The model under review builds one solid part; all positions refer to its coordinate system, in mm. Face numbers are marked on the shaded views. Coordinates: 2 decimals unless noted, no trailing zeros. Loops run counter-clockwise (first coordinate to the right, second up) from the corner with the lowest first, then second, coordinate; pieces in that order, holes last. Notation, with made-up numbers: (-22, -32) -> (13, -32) arc R14 ccw to (13, -17) -> close; hole circle Ø6 at (59, 15). An arc over 180 degrees is marked (long way). One line per question, with ' | ' between items. Start each with the question number.
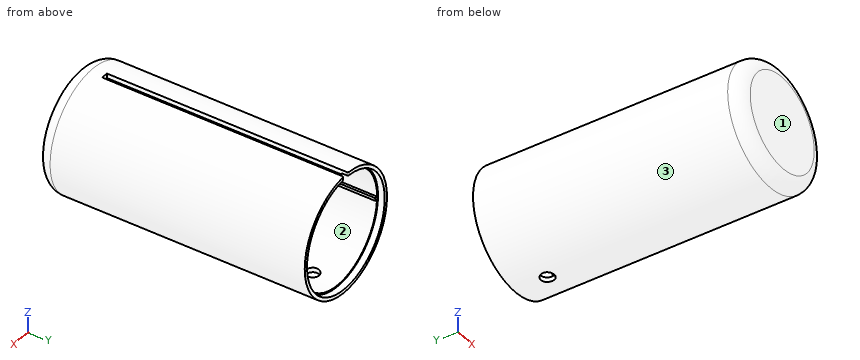
Autodesk Inventor part; units mm, degrees
ref_plane "Work Plane1" through (0, 200, -45) normal (0, 0, -1) x (-1, 0, 0)
ref_plane "YZ Plane" through (0, 0, 0) normal (1, 0, 0) x (0, 1, 0)
ref_plane "XZ Plane" through (0, 0, 0) normal (0, 1, 0) x (-1, 0, 0)
sketch "Sketch1" plane through (0, 0, 0) normal (0, 0, 1) x (1, 0, 0)
  line L0 (0, 0) -> (35, 0)
  line L1 (45, 10) -> (45, 200)
  line L2 (0, 200) -> (0, 0)
  arc A0 (35, 0) -> (45, 10) centre (35, 10) ccw
  line L3 (41.5, 200) -> (41.5, 10)
  arc A1 (35, 3.5) -> (41.5, 10) centre (35, 10) ccw
  line L4 (35, 3.5) -> (0, 3.5)
  line L5 (41.5, 200) -> (45, 200)
  line L6 (0, 3.5) -> (0, 0)
  point P0 (45, 0)
  dimension "d0" = 90
  dimension "d1" = 200
  dimension "d2" = 10
  dimension "d5" = 3.5
  dimension "d6" = 3.5
revolve "Revolution1" add sketch "Sketch1" angle 360 about axis through (0, 200, 0) along (0, -1, 0)
sketch "Sketch2" plane through (0, 200, 0) normal (0, 1, 0) x (1, 0, 0)
  circle A0 centre (0, 0) radius 45 construction
  line L0 (0, 45) -> (0, -45) construction
  line L1 (-45, 0) -> (45, 0) construction
  circle A1 centre (0, 0) radius 45 construction
  circle A2 centre (0, 0) radius 41.5 construction
  circle A3 centre (0, 0) radius 41.5 construction
  circle A4 centre (0, 0) radius 45 construction
  line L2 (0, -41.5) -> (0, -45) construction
  line L3 (-2.5, -45.45) -> (2.5, -45.45)
  line L4 (2.5, -45.45) -> (2.5, -41.05)
  line L5 (2.5, -41.05) -> (-2.5, -41.05)
  line L6 (-2.5, -41.05) -> (-2.5, -45.45)
  line L7 (-2.5, -45.45) -> (2.5, -41.05) construction
  line L8 (2.5, -45.45) -> (-2.5, -41.05) construction
  point P0 (0, -43.25)
  dimension "d8" = 5
  dimension "d9" = 4.4
extrude "Extrusion1" cut sketch "Sketch2" against normal blind 180
fillet "Fillet1" radius 1 2 edges at (-2.5, 200, 43.1776) (2.5, 200, 43.1776)
sketch "Sketch3" plane through (0, 200, 0) normal (0, 1, 0) x (1, 0, 0)
  arc A0 (3.5, -41.3521) -> (-3.5, -41.3521) centre (0, 0) ccw
  circle A1 centre (0, 0) radius 42.5
  circle A2 centre (0, 0) radius 41.5
  point P0 (3.5, -41.3521)
  point P1 (-3.5, -41.3521)
  dimension "d13" = 85
extrude "Extrusion2" cut sketch "Sketch3" against normal blind 5
ref_plane "Work Plane1" through (0, 200, -45) normal (0, 0, -1) x (-1, 0, 0)
sketch "Sketch4" plane through (0, 200, -45) normal (0, 0, -1) x (-1, 0, 0)
  line L0 (-45, 0) -> (45, 0) construction
  line L1 (0, 0) -> (0, -25) construction
  circle A0 centre (0, -25) radius 5
  point P0 (0, -200)
  point P1 (3.5, 0)
  point P2 (-3.5, 0)
  dimension "d16" = 25
  dimension "d17" = 10
extrude "Extrusion3" cut sketch "Sketch4" against normal up to surface
sketch "Sketch5" plane through (0, 195, 0) normal (0, 1, 0) x (1, 0, 0)
  line L0 (2.5, -42.4264) -> (2.5, -41.4246) construction
  arc A0 (2.5, -42.4264) -> (-2.5, -42.4264) centre (0, 0) ccw construction
  line L1 (-2.5, -41.4246) -> (-2.5, -42.4264) construction
  arc A1 (2.5, -41.4246) -> (-2.5, -41.4246) centre (0, 0) ccw
  arc A2 (2.5, -41.4246) -> (-2.5, -41.4246) centre (0, 0) ccw construction
  line L2 (41.5, 0) -> (-41.5, 0) construction
  line L3 (41.5, 0) -> (39.5, 0)
  arc A3 (39.5, 0) -> (39.4459, 2.0673) centre (0, 0) ccw
  line L4 (41.5, 0) -> (39.5, 0)
  line L5 (0, 0) -> (41.5, 0) construction
  line L6 (0, 0) -> (41.4431, 2.1719) construction
  line L7 (41.4431, 2.1719) -> (39.4459, 2.0673)
  line L8 (0, 41.5) -> (0, -41.5) construction
  arc A4 (41.5, 0) -> (41.4431, 2.1719) centre (0, 0) ccw
  arc A5 (-2.5, -41.4246) -> (2.5, -41.4246) centre (0, 0) ccw
  line L9 (-41.5, 0) -> (-39.5, 0)
  arc A6 (-39.4459, 2.0673) -> (-39.5, 0) centre (0, 0) ccw
  line L10 (-41.4431, 2.1719) -> (-39.4459, 2.0673)
  arc A7 (-41.4431, 2.1719) -> (-41.5, 0) centre (0, 0) ccw
  point P0 (-41.5, 0)
  dimension "d20" = 2
  dimension "d21" = 3
extrude "Extrusion4" add sketch "Sketch5" against normal blind 170 contours L3 A3 L7 A1 | A1 L10 A6 L9
properties part number "_3DPrint"
1) Consider section A-A, the plane x = 0. Write out the cut boundary in (y, z).
2) Consider section B-B, the plane y = 175. Write out the cut boundary in (x, z).
3) Consider section C-C, the plane y = 85. Write out the cut boundary in (x, z), plus the area to 3 significant figures.
4) Mouldability with a two-part tool opening along Z and no side actions: class the marked faces 1, 2 and 3 as +Z half, -Z half, draft (parallel to the pull), parting line (faces both ways), or undercut.
5) Insertion check: pin 1 Ø5 at (y, z) = (140.5, 31) entering from -X; pin 2 Ø4 at (y, z) = (113.5, -9.5) entering from +X; pin 3 Ø6 at (x, y) = (0, 175) entering from -Z; pin 4 Ø5 at (x, z) = (-29.5, -7.5) entering from -Y. Each pin has a flat end and moves straight along its axis. Give the tip position at first contact, or say it passes through.
6) Wall thickness on L1, parallel to Z at x = 2, y = 124; L2, parallel to Y at x = -4.5, z = 11; L3, parallel to Z at x = 35.5, y = 137.5: over which ranges is each line inside the solid? List them lowest first.
Filled sheet:
1) outline: (0, -35) arc R10 ccw to (10, -45) -> (170, -45) -> (170, -41.5) -> (10, -41.5) arc R6.5 cw to (3.5, -35) -> (3.5, 35) arc R6.5 cw to (10, 41.5) -> (20, 41.5) -> (20, 45) -> (10, 45) arc R10 ccw to (0, 35) -> close; (180, -45) -> (200, -45) -> (200, -42.5) -> (195, -42.5) -> (195, -41.5) -> (180, -41.5) -> close
2) outline: (-41.5, 0) arc R41.5 cw to (-2.5, 41.42) -> (-2.5, 44.93) arc R45 ccw to (-5, -44.72) -> (-5, -41.2) arc R41.5 cw to (-41.44, -2.17) -> (-39.45, -2.07) arc R39.45 cw to (-39.5, 0) -> close; (2.5, 41.42) arc R41.5 cw to (41.5, 0) -> (39.5, 0) arc R39.55 cw to (39.45, -2.07) -> (41.44, -2.17) arc R41.5 cw to (5, -41.2) -> (5, -44.72) arc R45 ccw to (2.5, 44.93) -> close
3) outline: (-41.5, 0) arc R41.5 cw to (-2.5, 41.42) -> (-2.5, 44.93) arc R45 ccw (long way) to (2.5, 44.93) -> (2.5, 41.42) arc R41.5 cw to (41.5, 0) -> (39.5, 0) arc R39.55 cw to (39.45, -2.07) -> (41.44, -2.17) arc R41.5 cw to (-41.44, -2.17) -> (-39.45, -2.07) arc R39.45 cw to (-39.5, 0) -> close | area: 942 mm^2
4) face 1: draft | face 2: undercut | face 3: parting line
5) pin 1: x = -34.82 | pin 2: x = 44.37 | pin 3: z = 41.39 | pin 4: y = 0
6) L1: -44.96 to -41.45 | L2: 0 to 3.5 | L3: -27.65 to -21.49, 21.49 to 27.65
